Build history of the part. All positions in model axes, mm. A direction names the side the tool comes from. Round coordinates to 2 decimals unless told otherwise and drop trailing zeros. Write each loop counter-clockwise with the first axis right and the second up, starting at its lowest first coordinate (ties: lowest second). Pieces come first, ordered by that corner, then holes.
Item 1: 3-axis set-ups, long thin cutter, end or side, ignore diameter. For faces 5 (the cylindrical face through (2.59, 1.06, -22.33)), 6 (the flat face through (2.5, -2.5, -22.3)), 7 (the flat face through (2.5, 2.5, -22.3)): which of +Z, -Z, +X, -X, +Y, -Y reach the whole face in a straight line?
Item 2: Mould opens along X. For faces 1 (the flat face through (-2.5, -2.5, -22.3)), 2 (the flat face through (-2.5, 2.5, -22.3)), 3 (the flat face through (4, -2, -5.588)), 4 (the cylindrical face through (-7.559, -5.796, -2.755)) say: +X half, -X half, draft (parallel to the pull), parting line (faces both ways), or undercut.
Item 3: Band-saw the part on B-B, the plane z = -5. Write the cut outline in (x, y) (3 decimals).
Item 4: Wall check: probe 1 along Y at (x, z) = (0, -16.5); probe 2 along Z at (x, y) = (5.25, -1.5); probe 3 along Z at (x, y) = (-0.25, 1.75). Give the ranges that are in metal, low to high.
Item 5: Band-saw the part on C-C, the plane x = 4. Write the cut outline in (y, z), then the cut area to 3 significant figures.
Item 6: Band-saw the part on D-D, the plane y = -7. Write the cut outline in (x, z), then the cut area to 3 significant figures.
Item 7: Drop flat-ended pins along their axis: pin 1 Ø5 at (y, z) = (5.5, -14) entering from +X; pin 2 Ø3 at (y, z) = (5.5, -9) entering from +X; pin 3 Ø8 at (y, z) = (-4, -17.5) entering from +X. Give the stop position or say it passes through.
Item 8: Band-saw the part on A-A, the plane x = 0.5. Write the cut outline in (y, z) (3 decimals), then the cut area to 3 significant figures.
```python
from build123d import *

# Parameters (mm, degrees)
SKETCH1_R           = 4.318
BOSS_EXTRUDE1_DEPTH = 21.082
SKETCH2_R           = 9.525
BOSS_EXTRUDE2_DEPTH = 5.588
BOSS_EXTRUDE3_DEPTH = 2.54
SKETCH6_R           = 1.55
CUT_EXTRUDE1_DEPTH  = 24.622


with BuildPart() as part:
    # Sketch1 → Boss-Extrude1 (new body)
    with BuildSketch(Plane.XY):
        Circle(SKETCH1_R)
    extrude(amount=-BOSS_EXTRUDE1_DEPTH)

    # Sketch2 → Boss-Extrude2 (add)
    with BuildSketch(Plane.XY):
        Circle(SKETCH2_R)
    extrude(amount=-BOSS_EXTRUDE2_DEPTH)

    # Sketch3 → Boss-Extrude3 (add)
    with BuildSketch(Plane(origin=(0, 0, -21.082), x_dir=(-1, 0, 0), z_dir=(0, 0, -1))):
        with BuildLine():
            Line((1.979898987, -1.979898987), (3.053287081, -3.053287081))
            ThreePointArc((3.053287081, -3.053287081), (3.989311821, -1.652427061), (4.318, 0))
            Line((4.318, 0), (2.8, 0))
            ThreePointArc((2.8, 0), (2.586862691, -1.071513611), (1.979898987, -1.979898987))
        make_face()
        with BuildLine():
            ThreePointArc((-3.053287081, 3.053287081), (-3.989311821, 1.652427061), (-4.318, 0))
            Line((-4.318, 0), (-2.8, 0))
            ThreePointArc((-2.8, 0), (-2.586862691, 1.071513611), (-1.979898987, 1.979898987))
            Line((-1.979898987, 1.979898987), (-3.053287081, 3.053287081))
        make_face()
        with BuildLine():
            ThreePointArc((-3.053287081, -3.053287081), (-1.652427061, -3.989311821), (0, -4.318))
            Line((0, -4.318), (0, -2.8))
            ThreePointArc((0, -2.8), (-1.071513611, -2.586862691), (-1.979898987, -1.979898987))
            Line((-1.979898987, -1.979898987), (-3.053287081, -3.053287081))
        make_face()
        with BuildLine():
            Line((0, 4.318), (0, 2.8))
            ThreePointArc((0, 2.8), (1.071513611, 2.586862691), (1.979898987, 1.979898987))
            Line((1.979898987, 1.979898987), (3.053287081, 3.053287081))
            ThreePointArc((3.053287081, 3.053287081), (1.652427061, 3.989311821), (0, 4.318))
        make_face()
    extrude(amount=BOSS_EXTRUDE3_DEPTH)

    # Sketch6 → Cut-Extrude1 (cut, through all)
    with BuildSketch(Plane.XY):
        Circle(SKETCH6_R)
    extrude(amount=-CUT_EXTRUDE1_DEPTH, mode=Mode.SUBTRACT)


solid = part.part
```
Results:
1. face 5: -Z, -X
1. face 6: -Z, +X
1. face 7: -Z, +Y
2. face 1: undercut
2. face 2: -X half
2. face 3: draft
2. face 4: parting line
3. outline: circle Ø19.05 at (0, 0); hole circle Ø3.1 at (0, 0)
4. probe 1: y = -4.32 to -1.55, 1.55 to 4.32
4. probe 2: z = -5.59 to 0
4. probe 3: z = -21.08 to 0
5. outline: (-8.64, -5.59) - (-1.63, -5.59) - (-1.63, -21.08) - (0, -21.08) - (0, -23.62) - (1.63, -23.62) - (1.63, -5.59) - (8.64, -5.59) - (8.64, 0) - (-8.64, 0) - close
5. area: 151 mm2
6. outline: (-6.46, -5.59) - (6.46, -5.59) - (6.46, 0) - (-6.46, 0) - close
6. area: 72.2 mm2
7. pin 1: stops at x = 3.11
7. pin 2: stops at x = 1.63
7. pin 3: stops at x = 4.32
8. outline: (-9.512, -5.588) - (-4.289, -5.588) - (-4.289, -23.622) - (-2.755, -23.622) - (-2.755, -21.082) - (-1.467, -21.082) - (-1.467, 0) - (-9.512, 0) - close; (1.467, -21.082) - (4.289, -21.082) - (4.289, -5.588) - (9.512, -5.588) - (9.512, 0) - (1.467, 0) - close
8. area: 181 mm2
